Here's how the part is built. I have some questions about the finished solid (model axes, mm). Round coordinates to 2 decimals unless told otherwise and drop trailing zeros. Write each loop counter-clockwise with the first axis right and the second up, starting at its lowest first coordinate (ties: lowest second). Pieces come first, ordered by that corner, then holes. Notation, with made-up numbers: (1.5, 27) -> (49.5, 27) arc R25 cw to (49.5, 58) -> close; hole circle Ø10 at (8.5, -34). An arc over 180 degrees is marked (long way). Answer in a Markdown table with one row per item.
from build123d import *

# Parameters (mm, degrees)
ESQUISSE1_R             = 22.2
BOSS_EXTRU_1_DEPTH      = 4.8
ESQUISSE2_R             = 3
ESQUISSE2_R_2           = 1.2
ENL_V_MAT_EXTRU_1_DEPTH = 32.760352643


with BuildPart() as part:
    # Esquisse1 → Boss.-Extru.1 (new body)
    with BuildSketch(Plane.XY):
        Circle(ESQUISSE1_R)
    extrude(amount=BOSS_EXTRU_1_DEPTH)

    # Esquisse2 → Enlèv. mat.-Extru.1 (cut, through all)
    with BuildSketch(Plane.XY.offset(4.8)):
        Circle(ESQUISSE2_R)
        with Locations((9.6, 0)):
            Circle(ESQUISSE2_R_2)
        with Locations((6.788225099, -6.788225099)):
            Circle(ESQUISSE2_R_2)
        with Locations((0, -9.6)):
            Circle(ESQUISSE2_R_2)
        with Locations((-6.788225099, -6.788225099)):
            Circle(ESQUISSE2_R_2)
        with Locations((-9.6, 0)):
            Circle(ESQUISSE2_R_2)
        with Locations((-6.788225099, 6.788225099)):
            Circle(ESQUISSE2_R_2)
        with Locations((0, 9.6)):
            Circle(ESQUISSE2_R_2)
        with Locations((6.788225099, 6.788225099)):
            Circle(ESQUISSE2_R_2)
        with BuildLine():
            Line((-13.996985601, 9.29109219), (-10.497739201, 6.968319142))
            ThreePointArc((-10.497739201, 6.968319142), (-7.916457842, 9.802535144), (-4.602380866, 11.729368711))
            Line((-4.602380866, 11.729368711), (-6.136507821, 15.639158282))
            ThreePointArc((-6.136507821, 15.639158282), (-10.555277122, 13.070046858), (-13.996985601, 9.29109219))
        make_face()
        with BuildLine():
            Line((1.047829065, 16.767291202), (0.785871799, 12.575468401))
            ThreePointArc((0.785871799, 12.575468401), (4.531015535, 11.757121171), (7.856740841, 9.850463103))
            Line((7.856740841, 9.850463103), (10.475654455, 13.133950804))
            ThreePointArc((10.475654455, 13.133950804), (6.041354047, 15.676161561), (1.047829065, 16.767291202))
        make_face()
        with BuildLine():
            Line((15.044814666, 7.476199012), (11.283610999, 5.607149259))
            ThreePointArc((11.283610999, 5.607149259), (12.447473377, 1.954586027), (12.459121707, -1.878905608))
            Line((12.459121707, -1.878905608), (16.612162276, -2.505207477))
            ThreePointArc((16.612162276, -2.505207477), (16.596631169, 2.606114703), (15.044814666, 7.476199012))
        make_face()
        with BuildLine():
            Line((13.996985601, -9.29109219), (10.497739201, -6.968319142))
            ThreePointArc((10.497739201, -6.968319142), (7.916457842, -9.802535144), (4.602380866, -11.729368711))
            Line((4.602380866, -11.729368711), (6.136507821, -15.639158282))
            ThreePointArc((6.136507821, -15.639158282), (10.555277122, -13.070046858), (13.996985601, -9.29109219))
        make_face()
        with BuildLine():
            Line((-1.047829065, -16.767291202), (-0.785871799, -12.575468401))
            ThreePointArc((-0.785871799, -12.575468401), (-4.531015535, -11.757121171), (-7.856740841, -9.850463103))
            Line((-7.856740841, -9.850463103), (-10.475654455, -13.133950804))
            ThreePointArc((-10.475654455, -13.133950804), (-6.041354047, -15.676161561), (-1.047829065, -16.767291202))
        make_face()
        with BuildLine():
            Line((-15.044814666, -7.476199012), (-11.283610999, -5.607149259))
            ThreePointArc((-11.283610999, -5.607149259), (-12.447473377, -1.954586027), (-12.459121707, 1.878905608))
            Line((-12.459121707, 1.878905608), (-16.612162276, 2.505207477))
            ThreePointArc((-16.612162276, 2.505207477), (-16.596631169, -2.606114703), (-15.044814666, -7.476199012))
        make_face()
    extrude(amount=-ENL_V_MAT_EXTRU_1_DEPTH, mode=Mode.SUBTRACT)


solid = part.part
1) I want a section at B-B, the plane x = 0. List the corners of the cut face in (y, z) for me.
Response:
| item | result |
|---|---|
| outline | (-22.2, 0) -> (-10.8, 0) -> (-10.8, 4.8) -> (-22.2, 4.8) -> close; (-8.4, 0) -> (-3, 0) -> (-3, 4.8) -> (-8.4, 4.8) -> close; (3, 0) -> (8.4, 0) -> (8.4, 4.8) -> (3, 4.8) -> close; (10.8, 0) -> (22.2, 0) -> (22.2, 4.8) -> (10.8, 4.8) -> close |
2) I need wall thicknesses on line 1 (Y direction, x = 0, z = 3.55); line 2 (Y direction, x = 9.6, z = 1.2); line 3 (Y direction, x = 11.5, z = 3.95). Which ranges of each line are inside material? Lowest first, please. Write a range as [from, to].
Response:
| item | result |
|---|---|
| line 1 | y = [-22.2, -10.8], [-8.4, -3], [3, 8.4], [10.8, 22.2] |
| line 2 | y = [-20.02, -13.79], [-8.16, -1.2], [1.2, 12.04], [13.79, 20.02] |
| line 3 | y = [-18.99, -12.25], [-7.63, 5.15], [5.71, 18.99] |
3) For pin 1 (1.9 mm diameter, centred on x = -9.6, y = 0, fed in from -Z); pin 2 (1 mm diameter, centred on x = -12.5, z = 2.5, fed in from -Y), each with a flat end and sliding along its axis, tell me the tip position at first contact or that it passes through.
Response:
| item | result |
|---|---|
| pin 1 | passes through |
| pin 2 | stops at y = -18.68 |
4) We'd pull the mould along Y, two halves only. Please class faces 1 (the face through (-4.481, -11.776, 2.434)), 2 (the face through (11.93, 18.72, 2.37)): +Y half, -Y half, draft (parallel to the pull), parting line (faces both ways), or undercut.
Response:
| item | result |
|---|---|
| face 1 | undercut |
| face 2 | parting line |
5) I want a section at A-A, the plane y = 0. List the corners of the cut face in (x, z) for me.
Response:
| item | result |
|---|---|
| outline | (-22.2, 0) -> (-16.8, 0) -> (-16.8, 4.8) -> (-22.2, 4.8) -> close; (-12.6, 0) -> (-10.8, 0) -> (-10.8, 4.8) -> (-12.6, 4.8) -> close; (-8.4, 0) -> (-3, 0) -> (-3, 4.8) -> (-8.4, 4.8) -> close; (3, 0) -> (8.4, 0) -> (8.4, 4.8) -> (3, 4.8) -> close; (10.8, 0) -> (12.6, 0) -> (12.6, 4.8) -> (10.8, 4.8) -> close; (16.8, 0) -> (22.2, 0) -> (22.2, 4.8) -> (16.8, 4.8) -> close |
6) I want a section at C-C, the plane z = 0.55. Count the separate pieces of the cut face and the enclosed holes in it, and give its area (3 significant figures).
Response:
| item | result |
|---|---|
| separate pieces | 1 |
| enclosed holes | 15 |
| area | 1,260 mm^2 |
7) I want a section at D-D, the plane x = -9.6. List the corners of the cut face in (y, z) for me, and give its area (3 significant figures).
Response:
| item | result |
|---|---|
| outline | (-20.02, 0) -> (-13.79, 0) -> (-13.79, 4.8) -> (-20.02, 4.8) -> close; (-12.04, 0) -> (-1.2, 0) -> (-1.2, 4.8) -> (-12.04, 4.8) -> close; (1.2, 0) -> (8.16, 0) -> (8.16, 4.8) -> (1.2, 4.8) -> close; (13.79, 0) -> (20.02, 0) -> (20.02, 4.8) -> (13.79, 4.8) -> close |
| area | 145 mm^2 |
